```python
from build123d import *

# Parameters (mm, degrees)
F1_DEPTH = 25.4
F2_DEPTH = 25.4
F4_DEPTH = 25.4
F5_DEPTH = 25.4


with BuildPart() as f1:
    # F0 (on Top) → F1 (new body)
    with BuildSketch(Plane.XY):
        Polygon((68.424131, 29.676452), (-7.079764, 74.245743), (-72.799666, 16.209941), (-37.912904, -64.227449), (49.368203, -55.904687), align=None)
    extrude(amount=F1_DEPTH)

    # F1_face (on face) → F2 (join)
    with BuildSketch(Plane(origin=(0, 0, 0), x_dir=(1, 0, 0), z_dir=(0, 0, -1))):
        Polygon((68.424131, -29.676452), (49.368203, 55.904687), (-37.912904, 64.227449), (-72.799666, -16.209941), (-7.079764, -74.245743), align=None)
    extrude(amount=F2_DEPTH)

    # F3 (on face) → F4 (cut)
    with BuildSketch(Plane.XY.offset(25.4)):
        Polygon((52.176996, 28.531717), (-11.011697, 58.440058), (-58.982599, 7.586225), (-25.441554, -53.751513), (43.258854, -40.806487), align=None)
    extrude(amount=-F4_DEPTH, mode=Mode.SUBTRACT)

    # F4_face (on face) → F5 (cut)
    with BuildSketch(Plane.XY):
        Polygon((52.176996, 28.531717), (-11.011697, 58.440058), (-58.982599, 7.586225), (-25.441554, -53.751513), (43.258854, -40.806487), align=None)
    extrude(amount=-F5_DEPTH, mode=Mode.SUBTRACT)


solid = f1.part
```
Work out the finished part from the listing and answer in its coordinate system (mm). A direction names the side the tool comes from. Give positions to 0.01 mm unless a question says otherwise; leave off trailing zeros. Loops run counter-clockwise (first coordinate to the right, second up) from the corner with the lowest first, then second, coordinate; pieces in that order, holes last. Notation, with made-up numbers: (67, 55) - (84, 55) arc R27 cw to (84, 74) - close; hole circle Ø8 at (17, -37.5). An arc over 180 degrees is marked (long way). Use CSV: the item, a comma, the result in double quotes. Start each with the question number.
(1) A tool of negligible diameter and unlimited length cuts with its end or side. For faces 5 (the face through (47.655, -6.623, 0.356)), 6 (the face through (-34, 35, -25.4)), from which of +Z, -Z, +X, -X, +Y, -Y can it reach the whole face along a straight path? Write none if from no direction.
(2) Find section C-C, the plane y = 25. Determine the outline of the cut face in (x, z).
(3) Find section B-B, the plane x = 38.5. Determine the outline of the cut face in (y, z), plus the area to 3 significant figures.
(4) Each of these flat-tipped pins is pushed along its axis until it touches: pin 1 (1.5 mm diameter, centred on x = 49.5, z = 12.5, fed in from -Y); pin 2 (10 mm diameter, centred on y = -38, z = 16, fed in from -X); pin 3 (10 mm diameter, centred on y = 36, z = -6, fed in from +X). Where does it stop, or does it pass through?
(5) Find section D-D, the plane x = 54. Determine the outline of the cut face in (y, z), plus the area to 3 significant figures.
(6) Determine the mould class of faces 1 (the face through (-42.45, -22.65, 0.36)), 2 (the face through (8.43, -47.37, 0.36)), 3 (the face through (30.1, 52.3, 0.4)), 4 (the face through (-39, -31, 25.4)) for opening direction X: released by +X, released by -X, zero draft, split by the parting line, or undercut.
(7) Find section A-A, the plane z = 2. Determine the outline of the cut face in (x, y), plus the area to 3 significant figures.
(8) Find the intervals of material crossed by L1, parallel to X at y = -21, z = 23.5; L2, parallel to X at y = 56, z = 16; L3, parallel to Y at x = -18, z = 17.5, in increasing order.
Results found:
1,face 5,"+Z, -Z"
1,face 6,"-Z, +X, -X, +Y, -Y"
2,outline,"(-62.85, -25.4) - (-42.56, -25.4) - (-42.56, 25.4) - (-62.85, 25.4) - close; (51.72, -25.4) - (67.38, -25.4) - (67.38, 25.4) - (51.72, 25.4) - close"
3,outline,"(-56.94, -25.4) - (-41.7, -25.4) - (-41.7, 25.4) - (-56.94, 25.4) - close; (35.01, -25.4) - (47.34, -25.4) - (47.34, 25.4) - (35.01, 25.4) - close"
3,area,"1,400 mm^2"
4,pin 1,"y = -55.96"
4,pin 2,"x = -51.46"
4,pin 3,"x = 66.18"
5,outline,"(-35.1, -25.4) - (38.19, -25.4) - (38.19, 25.4) - (-35.1, 25.4) - close"
5,area,"3,720 mm^2"
6,face 1,"undercut"
6,face 2,"undercut"
6,face 3,"released by +X"
6,face 4,"zero draft"
7,outline,"(-72.8, 16.21) - (-37.91, -64.23) - (49.37, -55.9) - (68.42, 29.68) - (-7.08, 74.25) - close; hole (-58.98, 7.59) - (-25.44, -53.75) - (43.26, -40.81) - (52.18, 28.53) - (-11.01, 58.44) - close"
7,area,"4,820 mm^2"
8,L1,"-56.66 to -43.35, 45.81 to 57.14"
8,L2,"-27.74 to -13.31, -5.86 to 23.83"
8,L3,"-62.33 to -52.35, 51.03 to 64.6"
